```python
from build123d import *

# Parameters (mm, degrees)
F2_SIZE  = 1.27
F4_START = 4.445
F3_W     = 10.16
F3_H     = 2.54
F4_DEPTH = 20.955


with BuildPart() as f1:
    # F0 (on Front) → F1 (revolve)
    with BuildSketch(Plane.XZ):
        with BuildLine():
            Line((3.2377406023, 3.556), (5.715, 3.556))
            ThreePointArc((5.715, 3.556), (3.2688625698, 5.8839526256), (0, 6.731))
            Line((0, 6.731), (0.0627406023, -9.144))
            Line((0.0627406023, -9.144), (3.2377406023, -9.144))
            Line((3.2377406023, -9.144), (3.2377406023, 3.556))
        make_face()
    revolve(axis=Axis((0.0313703012, 0, -1.2065), (0.0039521331, 0, -0.9999921903)))

    # F2
    f2_edges = [f1.edges().sort_by_distance(p)[0] for p in [
        (-3.11216, 0, -9.169096),
    ]]
    chamfer(f2_edges, length=F2_SIZE)

    # F3 (on Top) → F4 (cut)
    with BuildSketch(Plane.XY.offset(F4_START)):
        Rectangle(F3_W, F3_H)
    extrude(amount=F4_DEPTH, mode=Mode.SUBTRACT)


solid = f1.part
```
Input: part model. Units: mm. Frame: model coordinates. A direction names the side the tool comes from. Give positions to 0.01 mm unless a question says otherwise; leave off trailing zeros. Use a Markdown table: item, result.
Q1. Access query for faces 1 (the flat face through (0, -1.27, 5)), 2 (the conical face through (1.513, 2.842, -2.086)). Directions: +Z, -Z, +X, -X, +Y, -Y. A direction counts if a zero-diameter tool reaches every point of the face in a straight line with its end or side. Return the directions, or none.
Entries:
| item | result |
|---|---|
| face 1 | +Z, +X, -X |
| face 2 | -Z |
Q2. First-contact query: P1, Ø1.5, axis at y = 4, z = 1, coming from the +X side; P2, Ø1, axis at x = 0.5, z = 2.5, coming from the +Y side; P3, Ø2.5, axis at x = -1.5, z = 6, coming from the -Y side; P4, Ø1, axis at x = -3.5, y = -2, coming from the -Z side. Flat tips, straight axial feed; report the tip coordinate or a pass-through.
Entries:
| item | result |
|---|---|
| P1 | passes through |
| P2 | stops at y = 3.22 |
| P3 | stops at y = -4.54 |
| P4 | stops at z = 3.52 |
Q3. Ray query, probe 1 along Y at (x, z) = (3.5, 4.75); probe 2 along Y at (x, z) = (-1.5, 5.75); probe 3 along Z at (x, y) = (4.25, 0.25) (3 decimals). Return the intervals inside material, ascending. Write a range as from..to.
Entries:
| item | result |
|---|---|
| probe 1 | y = -3.23..-1.27, 1.27..3.23 |
| probe 2 | y = -3.12..-1.27, 1.27..3.12 |
| probe 3 | z = 3.556..4.445 |
